Could you check a few things on this model? Use its own coordinates, in mm. A direction names the side the tool comes from. Round coordinates to 2 decimals unless told otherwise and drop trailing zeros. Write each loop counter-clockwise with the first axis right and the second up, starting at its lowest first coordinate (ties: lowest second). Pieces come first, ordered by that corner, then holes. Notation, with made-up numbers: (68.5, 29) - (118.5, 29) arc R11 cw to (118.5, 47) - close; hole circle Ø1 at (56.5, 61). An arc over 180 degrees is marked (long way). Write each question's results on one line, items separated by ' | '. Start each with the question number.
(1) On a 3-axis mill with a long thin cutter (end or side, diameter ignored), from which of +Z, -Z, +X, -X, +Y, -Y can I reach the whole of each face in a straight line? I mean faces 4 (the cylindrical face through (41.53, 38.99, 4.39)), 5 (the flat face through (22, 16, 0)), 6 (the cylindrical face through (28.44, 39.01, 2.42)). Say none if no direction works.
(2) Thinking about a two-plate mould opening in X: for faces 1 (the flat face through (0, 25, -1)), 2 (the flat face through (27, 40, 1)), 3 (the cylindrical face through (16.42, 39.01, 2.56)), which applies, +X half, -X half, draft (parallel to the pull), parting line (faces both ways), or undercut?
(3) For P1, Ø5, axis at x = 13.5, y = 6, coming from the +Z side; P2, Ø1.5, axis at x = 5, z = 15, coming from the -Y side, each with a flat end and sliding along its axis, tell me the tip position at first contact or that it passes through.
(4) Imagine slicing it at B-B on z = 15.75. Write out the boundary of the cut face in (x, y).
(5) Imagine slicing it at C-C on x = 39. Write out the boundary of the cut face in (y, z), then the cut area to 3 significant figures.
(6) Please list where these lines run through material, in increasing order: line 1 (X direction, y = 39, z = 6); line 2 (Z direction, x = 18, y = 9.5); line 3 (Y direction, x = 13.5, z = -0.9). Write a range as [from, to].
(7) Imagine slicing it at D-D on x = 10. Write out the boundary of the cut face in (y, z).
(8) Imagine slicing it at A-A on y = 6. Write out the boundary of the cut face in (x, z), then the cut area to 3 significant figures.
```python
from build123d import *

# Parameters (mm, degrees)
EXTRUDE_1_DEPTH     = 45
SKETCH_2_R          = 5.1
SKETCH_2_R_2        = 1.6
CUT_EXTRUDE_1_DEPTH = 63.841069373
SKETCH_3_R          = 3
SKETCH_3_W          = 17
SKETCH_3_H          = 18
CUT_EXTRUDE_2_DEPTH = 62.587336361
FILLET_1_R          = 8.5


with BuildPart() as part:
    # ｽｹｯﾁ1 → ﾎﾞｽ - 押し出し1 (new body)
    with BuildSketch(Plane(origin=(0, 0, 0), x_dir=(0, 0, -1), z_dir=(1, 0, 0))):
        Polygon((-18, 40), (-18, 38), (0, 38), (0, 0), (2, 0), (2, 40), align=None)
    extrude(amount=EXTRUDE_1_DEPTH)

    # ｽｹｯﾁ2 → ｶｯﾄ - 押し出し1 (cut, through all)
    with BuildSketch(Plane.XY):
        with Locations((22.5, 25)):
            Circle(SKETCH_2_R)
        with Locations((13.5, 6)):
            Circle(SKETCH_2_R_2)
        with Locations((31.5, 6)):
            Circle(SKETCH_2_R_2)
    extrude(amount=-CUT_EXTRUDE_1_DEPTH, mode=Mode.SUBTRACT)

    # ｽｹｯﾁ3 → ｶｯﾄ - 押し出し2 (cut, through all)
    with BuildSketch(Plane.XZ.offset(-38)):
        with Locations(Location((6, 6, 0), (0, 0, 270))):
            Circle(SKETCH_3_R)
        with Locations(Location((39, 6, 0), (0, 0, 270))):
            Circle(SKETCH_3_R)
        with Locations((22.5, 9)):
            Rectangle(SKETCH_3_W, SKETCH_3_H)
    extrude(amount=-CUT_EXTRUDE_2_DEPTH, mode=Mode.SUBTRACT)

    # ﾌｨﾚｯﾄ1
    fillet_1_edges = [part.edges().sort_by_distance(p)[0] for p in [
        (31, 39, 0),
        (14, 39, 0),
    ]]
    fillet(fillet_1_edges, radius=FILLET_1_R - 0.0001)  # a hair under: the kernel refuses the full size


solid = part.part
```
Response:
1) face 4: +Y, -Y | face 5: +Z, +X, -X, -Y | face 6: +Z, +Y, -Y
2) face 1: -X half | face 2: draft | face 3: undercut
3) P1: z = 0 | P2: y = 38
4) outline: (0, 38) - (14, 38) - (14, 40) - (0, 40) - close; (31, 38) - (45, 38) - (45, 40) - (31, 40) - close
5) outline: (0, -2) - (40, -2) - (40, 3) - (38, 3) - (38, 0) - (0, 0) - close; (38, 9) - (40, 9) - (40, 18) - (38, 18) - close | area: 104 mm²
6) line 1: [0, 3], [9, 14.38], [30.62, 36], [42, 45] | line 2: [-2, 0] | line 3: [0, 4.4], [7.6, 40]
7) outline: (0, -2) - (40, -2) - (40, 18) - (38, 18) - (38, 0) - (0, 0) - close
8) outline: (0, -2) - (11.9, -2) - (11.9, 0) - (0, 0) - close; (15.1, -2) - (29.9, -2) - (29.9, 0) - (15.1, 0) - close; (33.1, -2) - (45, -2) - (45, 0) - (33.1, 0) - close | area: 77.2 mm²
